Could you check a few things on this model? Use its own coordinates, in mm. Face numbers are marked on the shaded views. A direction names the side the tool comes from. Round coordinates to 2 decimals unless told otherwise and drop trailing zeros. Write each loop counter-clockwise with the first axis right and the second up, starting at its lowest first coordinate (ties: lowest second). Pieces come first, ordered by that corner, then holes. Notation, with made-up numbers: (47, 67) - (74, 67) arc R11 cw to (74, 85) - close; hole circle Ø2 at (-35.5, 13). An arc over 180 degrees is marked (long way). Put each result on its own line as item: value.
from build123d import *

# Parameters (mm, degrees)
SKETCH_2_R          = 1.5
CUT_EXTRUDE_1_DEPTH = 5
EXTRUDE_1_DEPTH     = 5
FILLET_1_R          = 0.5


with BuildPart() as part:
    # 草图1 → 旋转1 (revolve)
    with BuildSketch(Plane.XY):
        Polygon((0, 0), (0, 5), (25, 5), (25, 7.5), (30, 7.5), (30, 4), (55, 4), (55, 0), align=None)
    revolve(axis=Axis((0, 0, 0), (1, 0, 0)))

    # 草图2 → 切除-拉伸1 (cut, symmetric)
    with BuildSketch(Plane(origin=(0, 0, 0), x_dir=(1, 0, 0), z_dir=(0, 1, 0))):
        with Locations((5, 0)):
            Circle(SKETCH_2_R)
    extrude(amount=CUT_EXTRUDE_1_DEPTH, both=True, mode=Mode.SUBTRACT)

    # 草图3 → 凸台-拉伸1 (add)
    with BuildSketch(Plane(origin=(55, 0, 0), x_dir=(0, 0, -1), z_dir=(1, 0, 0))):
        Polygon((-2.757308573, 2.742691427), (-2.742691427, -2.757308573), (2.757308573, -2.742691427), (2.742691427, 2.757308573), align=None)
    extrude(amount=EXTRUDE_1_DEPTH)

    # 圆角1
    fillet_1_edges = [part.edges().sort_by_distance(p)[0] for p in [
        (57.5, 2.757308573, -2.742691427),
        (57.5, 2.742691427, 2.757308573),
        (57.5, -2.757308573, 2.742691427),
        (57.5, -2.742691427, -2.757308573),
    ]]
    fillet(fillet_1_edges, radius=FILLET_1_R)


solid = part.part
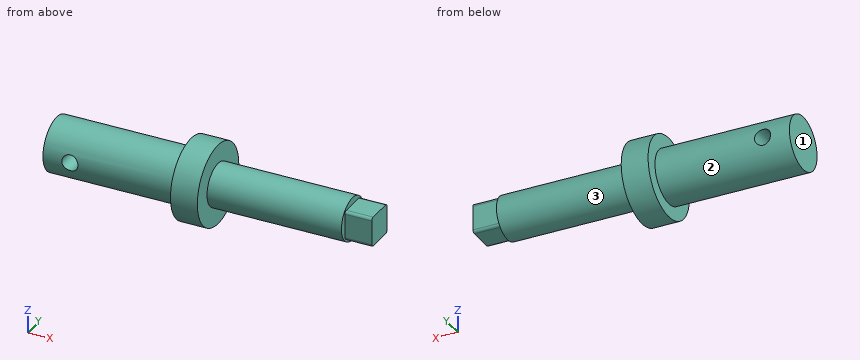
(1) I'm going to push flat-ended pins straight in: pin 1 (2 mm diameter, centred on x = 27, z = -2.5, fed in from +Y); pin 2 (1.5 mm diameter, centred on x = 17.5, y = -3, fed in from +Z); pin 3 (4 mm diameter, centred on x = 50, z = -1, fed in from -Y). Where does each tip first touch, or does it pass through?
Values found:
pin 1: stops at y = 7.35
pin 2: stops at z = 4.47
pin 3: stops at y = -4
(2) Imagine slicing it at C-C, the plane x = 13. List the corners of the cut face in (y, z) for me.
Values found:
outline: circle Ø10 at (0, 0)
(3) For the marked faces 1, 2 and 3, which set-ups out of +Z, -Z, +X, -X, +Y, -Y let a thin tool reach every point of the face, with its end or its side?
Values found:
face 1: +Z, -Z, -X, +Y, -Y
face 2: -X
face 3: +X
(4) Imagine slicing it at B-B, the plane z = 0. List the corners of the cut face in (x, y) for me.
Values found:
outline: (0, -5) - (3.5, -5) - (3.5, 5) - (0, 5) - close; (6.5, -5) - (25, -5) - (25, -7.5) - (30, -7.5) - (30, -4) - (55, -4) - (55, -2.75) - (60, -2.75) - (60, 2.75) - (55, 2.75) - (55, 4) - (30, 4) - (30, 7.5) - (25, 7.5) - (25, 5) - (6.5, 5) - close
(5) Please list where these lines run through material, in increasing order: probe 1 along X at (y, z) = (-1.75, 0); probe 2 along X at (y, z) = (-5.5, -3); probe 3 along X at (y, z) = (-2, 4.5). Write a range as from..to.
Values found:
probe 1: x = 0..3.5, 6.5..60
probe 2: x = 25..30
probe 3: x = 0..30
(6) Imagine slicing it at D-D, the plane x = 5. List the corners of the cut face in (y, z) for me, then the cut area to 3 significant figures.
Values found:
outline: (-4.77, -1.5) arc R5 ccw to (4.77, -1.5) - close; (-4.77, 1.5) - (4.77, 1.5) arc R5 ccw to start
area: 49.0 mm^2
(7) Imagine slicing it at A-A, the plane y = 0. List the corners of the cut face in (x, z) for me.
Values found:
outline: (0, -5) - (25, -5) - (25, -7.5) - (30, -7.5) - (30, -4) - (55, -4) - (55, -2.75) - (60, -2.75) - (60, 2.75) - (55, 2.75) - (55, 4) - (30, 4) - (30, 7.5) - (25, 7.5) - (25, 5) - (0, 5) - close; hole circle Ø3 at (5, 0)
